The drawing under review shows one solid part. Ordinate dimensions are in mm from its lowest x, y, z. Coordinates: 2 decimals unless noted, no trailing zeros. Write each loop counter-clockwise with the first axis right and the second up, starting at its lowest first coordinate (ties: lowest second). Pieces come first, ordered by that corner, then holes. Notation, with made-up numbers: (74, 66) - (129, 66) arc R22 cw to (129, 96) - close; hole circle Ø9 at (86.5, 40). An arc over 180 degrees is marked (long way). Use a Markdown table: item, result.
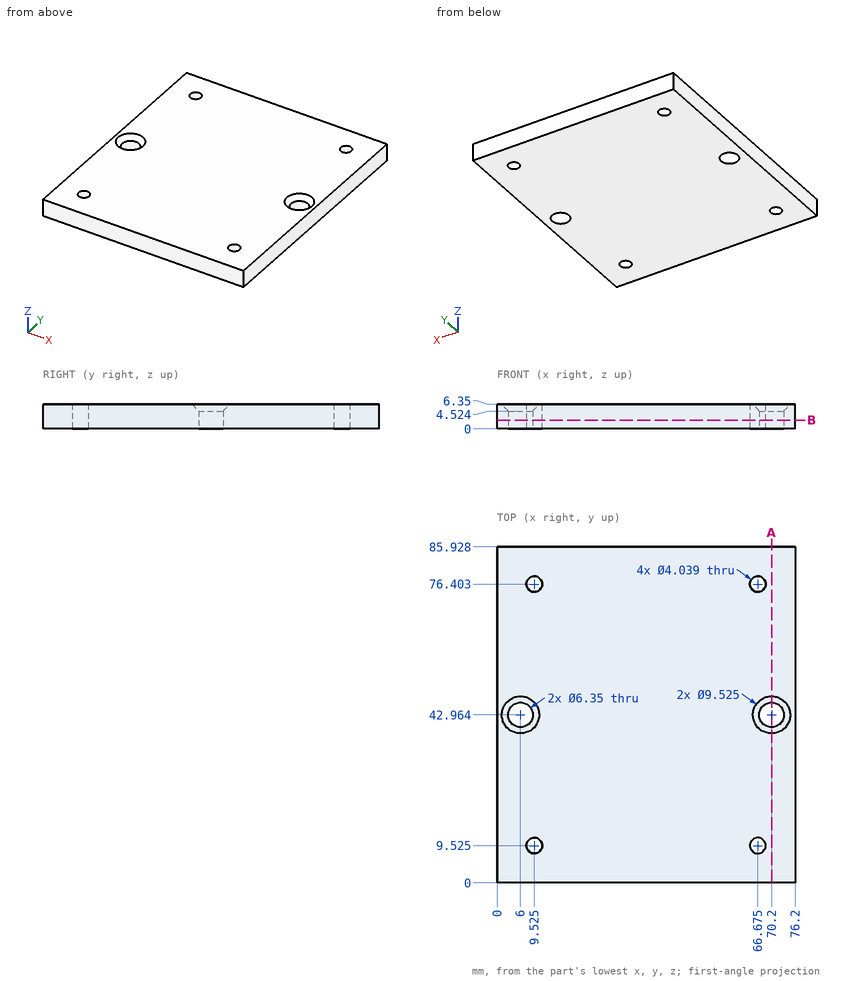
(1) Take a section at A-A on x = 70.2. Write out the cut boundary in (y, z).
Determined:
| item | result |
|---|---|
| outline | (0, 0) - (39.79, 0) - (39.79, 4.52) - (38.2, 6.35) - (0, 6.35) - close; (46.14, 0) - (85.93, 0) - (85.93, 6.35) - (47.73, 6.35) - (46.14, 4.52) - close |
(2) For L1, parallel to X at y = 76.5, z = 4.5; L2, parallel to Y at x = 70.2, z = 3.15; L3, parallel to Y at x = 67, z = 6 (1 decimal), list the stretches that pass through material, from the lowest coordinate up. Write a range as from..to.
Determined:
| item | result |
|---|---|
| L1 | 0..7.51, 11.54..64.66, 68.69..76.2 |
| L2 | 0..39.79, 46.14..85.93 |
| L3 | 0..7.5, 11.5..39.9, 46.1..74.4, 78.4..85.9 |
(3) Take a section at B-B on z = 2.25. State how many separate pieces and enclosed holes the cut face has, and give its area (3 significant figures).
Determined:
| item | result |
|---|---|
| separate pieces | 1 |
| enclosed holes | 6 |
| area | 6,430 mm2 |
